Autodesk Inventor part; units mm, degrees
ref_plane "Pracovní rovina1" through (0, 22, 0) normal (0, 1, 0) x (1, 0, 0)
ref_plane "YZ Plane" through (0, 0, 0) normal (1, 0, 0) x (0, 1, 0)
ref_plane "XZ Plane" through (0, 0, 0) normal (0, 1, 0) x (-1, 0, 0)
sketch "Náčrt1" plane through (0, 0, 0) normal (0, 1, 0) x (-1, 0, 0)
  circle A0 centre (0, 0) radius 92
  dimension "d0" = 184
extrude "Vysunutí1" add sketch "Náčrt1" along normal blind 2
sketch "Náčrt2" plane through (0, 2, 0) normal (0, 1, 0) x (1, 0, 0)
  circle A0 centre (0, 0) radius 86
  circle A1 centre (0, 0) radius 92
  dimension "d3" = 184
  dimension "d8" = 172
extrude "Vysunutí2" add sketch "Náčrt2" along normal blind 30
ref_plane "Pracovní rovina1" through (0, 22, 0) normal (0, 1, 0) x (1, 0, 0)
sketch "Náčrt3" plane through (0, 22, 0) normal (0, 1, 0) x (1, 0, 0)
  circle A0 centre (0, 0) radius 88.5
  dimension "d7" = 177
extrude "Vysunutí3" cut sketch "Náčrt3" along normal blind 5.1
sketch "Náčrt4" plane through (0, 32, 0) normal (0, 1, 0) x (1, 0, 0)
  circle A0 centre (0, 0) radius 88.5
  line L0 (-88.4633, 2.55) -> (-84.4633, 2.55)
  line L1 (-84.4633, 2.55) -> (-84.4633, -2.55)
  line L2 (-84.4633, -2.55) -> (-88.4633, -2.55)
  line L3 (-88.4633, -2.55) -> (-88.4633, 2.55)
  line L4 (0, 128.8) -> (0, -128.8)
  line L5 (128.8, 0) -> (-128.8, 0)
  line L6 (84.4633, 2.55) -> (88.4633, 2.55)
  line L7 (88.4633, 2.55) -> (88.4633, -2.55)
  line L8 (88.4633, -2.55) -> (84.4633, -2.55)
  line L9 (84.4633, -2.55) -> (84.4633, 2.55)
  dimension "d11" = 4
  dimension "d12" = 5.1
  dimension "d15" = 360
extrude "Vysunutí4" cut sketch "Náčrt4" against normal blind 5.1 contours L7 L5 L9 L6 | L8 L9 L5 L7 | L0 L1 L5 L3 | L3 L5 L1 L2
fillet "Zaoblení1" radius 10 1 edges at (92, 0, 0)
properties part number "Poklop"
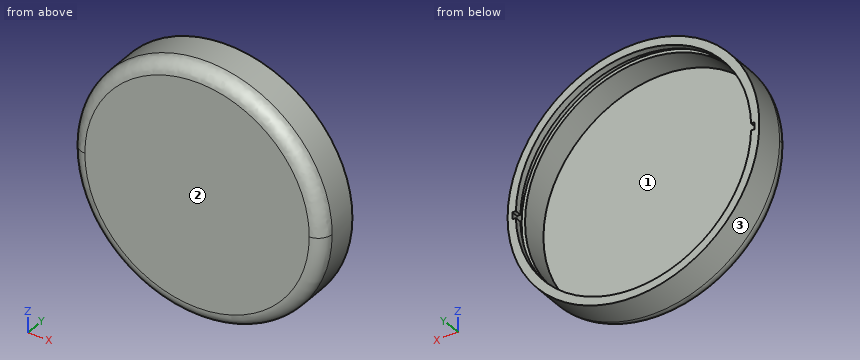
Read the model definition and answer for the solid it produces. Units are mm, in the model's axes. Face numbers are marked on the shaded views. Coordinates: 2 decimals unless noted, no trailing zeros. Order: outer loops, then holes, each group sorted by start corner. A loop starts at its lowest first (then second) coordinate and runs counter-clockwise, first axis right, second up. Notation, with made-up numbers: (-7.5, -13.5) - (1.5, -13.5) arc R15 cw to (1.5, 8.5) - close; hole circle Ø9 at (-36, -14.75). An arc over 180 degrees is marked (long way). Answer as a JSON object with one key per item and string values. Group by question number.
Item 1: Consider probe 1 along Z at (x, y) = (0, 23); probe 2 along Z at (x, y) = (0, 16); probe 3 along X at (y, z) = (9.25, 0). Determine where each line is inside the solid, lowest interval first. Write a range as from..to.
Item 2: Flat-ended cylindrical pins translate along their axes: P1, Ø10, axis at x = 10.5, y = 18.5, coming from the +Z side; P2, Ø5, axis at y = 16, z = -62, coming from the -X side; P3, Ø4, axis at x = -24.5, z = 37, coming from the +Y side. Find the tip coordinate at first contact, or state that the pin passes through.
Item 3: Section A-A (y = 17.5) is taken. Give the vertices of the cut face in (x, z), plus the area to 3 significant figures.
Item 4: The mould has two halves that part along Z. Classify the marked faces 1, 2 and 3: +Z half, -Z half, draft (parallel to the pull), parting line (faces both ways), or undercut.
Results are:
{
 "1": {"probe 1": "z = -92..-88.5, 88.5..92", "probe 2": "z = -92..-86, 86..92", "probe 3": "x = -91.97..-86, 86..91.97"},
 "2": {"P1": "stops at z = 91.84", "P2": "stops at x = -70.17", "P3": "stops at y = 2"},
 "3": {"outline": "circle Ø184 at (0, 0); hole circle Ø172 at (0, 0)", "area": "3,360 mm^2"},
 "4": {"face 1": "undercut", "face 2": "draft", "face 3": "parting line"}
}
